Can you work these out from the model? Positions are in its coordinate system, mm. A direction names the side the tool comes from. Round coordinates to 2 decimals unless told otherwise and drop trailing zeros. Loops run counter-clockwise (first coordinate to the right, second up) from the corner with the lowest first, then second, coordinate; pieces in that order, holes last.
```python
from build123d import *

# Parameters (mm, degrees)
F2_R     = 2.5
F3_DEPTH = 10


with BuildPart() as f1:
    # F0 (on Front) → F1 (revolve)
    with BuildSketch(Plane.XZ):
        Polygon((3, 10), (1, 8), (-1, 8), (-3, 10), (-5, 10), (-5, 0), (5, 0), (5, 10), align=None)
    revolve(axis=Axis((0, 0, 0), (1, 0, 0)))

    # F2 (on face) → F3 (cut, through all)
    with BuildSketch(Plane(origin=(-5, 0, 0), x_dir=(0, -1, 0), z_dir=(-1, 0, 0))):
        Circle(F2_R)
    extrude(amount=-F3_DEPTH, mode=Mode.SUBTRACT)


solid = f1.part
```
(1) For pin 1 (1.5 mm diameter, centred on x = -0.5, y = -3, fed in from +Z); pin 2 (3 mm diameter, centred on x = -3.5, y = -4, fed in from -Z), each with a flat end and sliding along its axis, tell me the tip position at first contact or that it passes through.
(2) Suppose I cut it at A-A (z = 0). Write out the boundary of the cut face in (x, y).
(3) If I drill on line 1 (Z direction, x = -0.5, y = 0); line 2 (Y direction, x = 4, z = -2.25); line 3 (Z direction, x = -1.5, y = 0), over which ranges is the centre line in solid material (lowest first)?
(4) Which directions (+Z, -Z, +X, -X, +Y, -Y) give clear straight access to the entire face, cutting with the end or side of a thin tool? Please do faces 4 (the cylindrical face through (3.99, 9.76, -2.17)), 5 (the conical face through (-1.13, -8.06, -1.06)).
(5) We'd pull the mould along Y, two halves only. Please class faces 1 (the cylindrical face through (-0.07, 0.54, -2.44)), 2 (the flat face through (-5, 2, 2)), 3 (the cylindrical face through (-4.01, 9.76, -2.17)): released by +Y, released by -Y, zero draft, split by the parting line, or undercut.
Check result:
1. pin 1: stops at z = 7.73
1. pin 2: stops at z = -9.68
2. outline: (-5, -10) - (-3, -10) - (-1, -8) - (1, -8) - (3, -10) - (5, -10) - (5, -2.5) - (-5, -2.5) - close; (-5, 2.5) - (5, 2.5) - (5, 10) - (3, 10) - (1, 8) - (-1, 8) - (-3, 10) - (-5, 10) - close
3. line 1: z = -8 to -2.5, 2.5 to 8
3. line 2: y = -9.74 to -1.09, 1.09 to 9.74
3. line 3: z = -8.5 to -2.5, 2.5 to 8.5
4. face 4: +X, -X
4. face 5: none
5. face 1: undercut
5. face 2: zero draft
5. face 3: split by the parting line
